Verification items for the finished model (mm, model axes). Face numbers are marked on the shaded views. A direction names the side the tool comes from. Give positions to 0.01 mm unless a question says otherwise; leave off trailing zeros. Answer as a JSON object with one key per item and string values. Group by question number.
Item 1: Scan lines: line 1 along Z through (x, y) = (50, 1.3); line 2 along X through (y, z) = (10.5, 1.5); line 3 along X through (y, z) = (80.5, -0.25). Record each from-to range of solid material in increasing order. Write a range as [from, to].
Item 2: Sectioned sample at A-A, the plane y = 36. Count the separate pieces of the cut face and the enclosed holes in it, and give its area (3 significant figures).
Item 3: Tool access check on the marked faces 1 and 2. Record the directions out of +Z, -Z, +X, -X, +Y, -Y that give a thin tool (end or side, any length) a straight path to the whole face; none if there is none.
Item 4: Go/stop test with flat-tipped pins: pin 1 (5 mm diameter, centred on y = 18, z = 2, fed in from +X); pin 2 (1.5 mm diameter, centred on x = -9, y = 15.5, fed in from +Z); pin 3 (3 mm diameter, centred on y = 2.5, z = 3, fed in from -X); pin 4 (3 mm diameter, centred on x = -50, z = 5, fed in from +Y). Record where each tip stops, or that it passes through.
Item 5: Draft check along X on the marked faces 3 and 4. Enter one of: +X half, -X half, draft (parallel to the pull), parting line (faces both ways), or undercut.
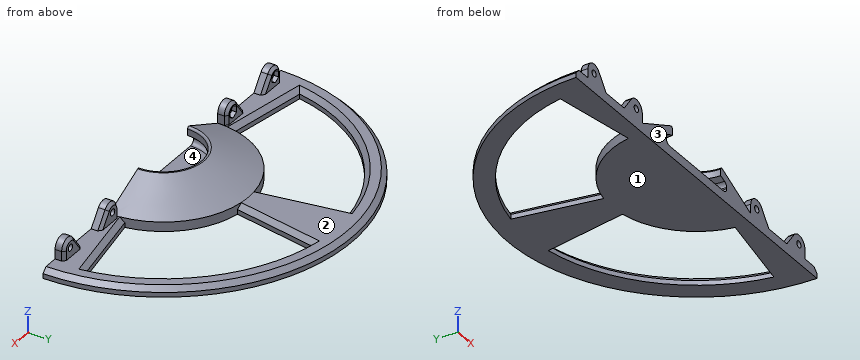
```python
from build123d import *

# Parameters (mm, degrees)
F1_ANGLE      = 180
F0_W          = 10
F0_H          = 5
F2_R          = 1
F3_R          = 2.5
F4_W          = 45
F4_H          = 5
F5_ANGLE      = 10
F6_W          = 45
F6_H          = 5
F7_ANGLE      = 10
F8_W          = 45
F8_H          = 5
F9_ANGLE_BACK = 10
F9_ANGLE      = 20
F10_R         = 1.75
F11_DEPTH     = 5
F13_DEPTH     = 2.5
F14_SIZE      = 2.5
F16_DEPTH     = 5
F17_SIZE      = 1.5


with BuildPart() as f1:
    # F0 (on Front) → F1 (revolve)
    with BuildSketch(Plane.XZ):
        Polygon((25, 0), (0, 0), (0, -5), (45, -5), (45, 0), (20, 11.8198511713), (20, 6.8198511713), (25, 5), align=None)
    revolve(axis=Axis((0, 0, -2.5), (0, 0, 1)), revolution_arc=F1_ANGLE)

    # F2
    f2_edges = [f1.edges().sort_by_distance(p)[0] for p in [
        (0, 20, 11.819851),
    ]]
    fillet(f2_edges, radius=F2_R)

    # F3
    f3_edges = [f1.edges().sort_by_distance(p)[0] for p in [
        (0, 25, 5),
        (0, 25, 0),
    ]]
    fillet(f3_edges, radius=F3_R)



with BuildPart() as f1b:
    # F0 (on Front) → F1, piece 2 (revolve)
    with BuildSketch(Plane.XZ):
        with Locations((95, -2.5)):
            Rectangle(F0_W, F0_H)
    revolve(axis=Axis((0, 0, -2.5), (0, 0, 1)), revolution_arc=F1_ANGLE)


with BuildPart() as f1_1:
    add(f1.part)

    add(f1b.part)  # F5 merges F1b
    # F4 (on face) → F5 (revolve)
    with BuildSketch(Plane.XZ):
        with Locations((67.5, -2.5)):
            Rectangle(F4_W, F4_H)
    revolve(axis=Axis((0, 0, 10), (0, 0, 1)), revolution_arc=F5_ANGLE)

    # F6 (on face) → F7 (revolve)
    with BuildSketch(Plane.XZ):
        with Locations((-67.5, -2.5)):
            Rectangle(F6_W, F6_H)
    revolve(axis=Axis((0, 0, 10), (0, 0, -1)), revolution_arc=F7_ANGLE)

    # F8 (on Right) → F9 (revolve)
    with BuildSketch(Plane.YZ, mode=Mode.PRIVATE) as f9_sk:
        with Locations((67.5, -2.5)):
            Rectangle(F8_W, F8_H)
    revolve(f9_sk.sketch.rotate(Axis((0, 0, 10), (0, 0, 1)), -F9_ANGLE_BACK), axis=Axis((0, 0, 10), (0, 0, 1)), revolution_arc=F9_ANGLE)

    # F10 (on face) → F11 (join)
    with BuildSketch(Plane.XZ):
        with BuildLine():
            Line((-90, 5), (-90, 0))
            Line((-90, 0), (-80, 0))
            Line((-80, 0), (-80, 5))
            ThreePointArc((-80, 5), (-85, 10), (-90, 5))
        make_face()
        with Locations((-85, 5)):
            Circle(F10_R, mode=Mode.SUBTRACT)
        with BuildLine():
            Line((-55, 0), (-45, 0))
            Line((-45, 0), (-45, 5))
            ThreePointArc((-45, 5), (-50, 10), (-55, 5))
            Line((-55, 5), (-55, 0))
        make_face()
        with Locations((-50, 5)):
            Circle(F10_R, mode=Mode.SUBTRACT)
        with BuildLine():
            Line((80, 5), (80, 0))
            Line((80, 0), (90, 0))
            Line((90, 0), (90, 5))
            ThreePointArc((90, 5), (85, 10), (80, 5))
        make_face()
        with Locations((85, 5)):
            Circle(F10_R, mode=Mode.SUBTRACT)
        with BuildLine():
            Line((45, 0), (55, 0))
            Line((55, 0), (55, 5))
            ThreePointArc((55, 5), (50, 10), (45, 5))
            Line((45, 5), (45, 0))
        make_face()
        with Locations((50, 5)):
            Circle(F10_R, mode=Mode.SUBTRACT)
    extrude(amount=-F11_DEPTH)

    # F12 (on face) → F13 (cut)
    with BuildSketch(Plane(origin=(0, 5, 0), x_dir=(-1, 0, 0), z_dir=(0, 1, 0))):
        Polygon((52.75, 3.4122867597), (52.75, 6.5877132403), (50, 8.1754264805), (47.25, 6.5877132403), (47.25, 3.4122867597), (50, 1.8245735195), align=None)
        Polygon((82.25, 6.5877132403), (82.25, 3.4122867597), (85, 1.8245735195), (87.75, 3.4122867597), (87.75, 6.5877132403), (85, 8.1754264805), align=None)
    extrude(amount=-F13_DEPTH, mode=Mode.SUBTRACT)

    # F14
    f14_edges = [f1_1.edges().sort_by_distance(p)[0] for p in [
        (-11.721252, 66.474523, 0),
        (11.721252, 66.474523, 0),
        (-63.63961, 63.63961, 0),
        (-66.474523, 11.721252, 0),
        (66.474523, 11.721252, 0),
        (63.63961, 63.63961, 0),
        (0, 100, 0),
    ]]
    chamfer(f14_edges, length=F14_SIZE)

    # F15 (on face) → F16 (join, through all)
    with BuildSketch(Plane.XZ):
        with BuildLine():
            Line((-80, 0), (-75, 0))
            Line((-75, 0), (-81, 8))
            ThreePointArc((-81, 8), (-80.2565835097, 6.5811388301), (-80, 5))
            Line((-80, 5), (-80, 0))
        make_face()
        with BuildLine():
            Line((-60, 0), (-55, 0))
            Line((-55, 0), (-55, 5))
            ThreePointArc((-55, 5), (-54.7434164903, 6.5811388301), (-54, 8))
            Line((-54, 8), (-60, 0))
        make_face()
        with BuildLine():
            ThreePointArc((54, 8), (54.7434164903, 6.5811388301), (55, 5))
            Line((55, 5), (55, 0))
            Line((55, 0), (60, 0))
            Line((60, 0), (54, 8))
        make_face()
        with BuildLine():
            Line((80, 0), (80, 5))
            ThreePointArc((80, 5), (80.2565835097, 6.5811388301), (81, 8))
            Line((81, 8), (75, 0))
            Line((75, 0), (80, 0))
        make_face()
    extrude(amount=-F16_DEPTH)

    # F17
    f17_edges = [f1_1.edges().sort_by_distance(p)[0] for p in [
        (-57, 5, 4),
        (-78, 5, 4),
        (78, 5, 4),
        (57, 5, 4),
        (90, 5, 2.5),
        (86.581139, 5, 9.743416),
        (48.418861, 5, 9.743416),
        (45, 5, 2.5),
        (-45, 5, 2.5),
        (-48.418861, 5, 9.743416),
        (-86.581139, 5, 9.743416),
        (-90, 5, 2.5),
    ]]
    chamfer(f17_edges, length=F17_SIZE)


solid = f1_1.part
```
Geometry check:
{
 "1": {"line 1": "[-5, 3.25], [6.75, 10]", "line 2": "[-40.49, -22.46], [22.46, 40.49]", "line 3": "[-55.45, -45.05], [-11.91, 11.91], [45.05, 55.45]"},
 "2": {"separate pieces": "3", "enclosed holes": "0", "area": "514 mm^2"},
 "3": {"face 1": "-Z, +X, -X, +Y, -Y", "face 2": "+Z, +Y"},
 "4": {"pin 1": "x = 96.37", "pin 2": "z = 0", "pin 3": "x = -90", "pin 4": "through"},
 "5": {"face 3": "draft", "face 4": "undercut"}
}
